Check sheet for the modelled part. Datum: model origin and axes. Units: mm. A direction names the side the tool comes from. Give positions to 0.01 mm unless a question says otherwise; leave off trailing zeros. Order: outer loops, then holes, each group sorted by start corner. A loop starts at its lowest first (then second) coordinate and runs counter-clockwise, first axis right, second up.
from build123d import *

# Parameters (mm, degrees)
F0_R     = 33
F1_DEPTH = 101.6
F2_R     = 26.5
F3_DEPTH = 76.2
F4_R     = 16
F5_DEPTH = 2
F6_R     = 6
F7_DEPTH = 26


with BuildPart() as f1:
    # F0 (on Right) → F1 (new body)
    with BuildSketch(Plane.YZ):
        Circle(F0_R)
    extrude(amount=F1_DEPTH)

    # F2 (on face) → F3 (join)
    with BuildSketch(Plane.YZ.offset(101.6)):
        Circle(F2_R)
    extrude(amount=F3_DEPTH)

    # F4 (on face) → F5 (join)
    with BuildSketch(Plane.YZ.offset(177.8)):
        Circle(F4_R)
    extrude(amount=F5_DEPTH)

    # F6 (on face) → F7 (join)
    with BuildSketch(Plane.YZ.offset(179.8)):
        Circle(F6_R)
    extrude(amount=F7_DEPTH)


solid = f1.part
1) Depth check by flat-ended pin: pin 1 Ø1.5 at (y, z) = (-22.5, 13) entering from +X; pin 2 Ø8 at (x, y) = (110, 3.5) entering from -Z; pin 3 Ø10 at (x, z) = (63, 18.5) entering from +Y. Enter the tip coordinate at first touch or a pass-through.
Recorded:
pin 1: stops at x = 177.8
pin 2: stops at z = -26.5
pin 3: stops at y = 30.11
2) Set-up check for faces 1 (the face through (139.167, 14.246, 22.345)), 2 (the face through (50.1, 30.5, -12.6)): record each of +Z, -Z, +X, -X, +Y, -Y from which the full face is reachable in a straight line by a thin tool's end or side.
Recorded:
face 1: +X
face 2: +X, -X
3) Section check A-A, the plane z = 0. Record the cut outline in (x, y), then the cut area to 3 significant figures.
Recorded:
outline: (0, -33) - (101.6, -33) - (101.6, -26.5) - (177.8, -26.5) - (177.8, -16) - (179.8, -16) - (179.8, -6) - (205.8, -6) - (205.8, 6) - (179.8, 6) - (179.8, 16) - (177.8, 16) - (177.8, 26.5) - (101.6, 26.5) - (101.6, 33) - (0, 33) - close
area: 11,100 mm2
4) Section check D-D, the plane y = -21. Record the cut outline in (x, z), then the cut area to 3 significant figures.
Recorded:
outline: (0, -25.46) - (101.6, -25.46) - (101.6, -16.16) - (177.8, -16.16) - (177.8, 16.16) - (101.6, 16.16) - (101.6, 25.46) - (0, 25.46) - close
area: 7,640 mm2
5) Material ranges on L1, parallel to X at y = 17.5, z = -1; L2, parallel to X at y = -1.5, z = 10.5; L3, parallel to Z at x = 69, y = 1, recorded low to high.
Recorded:
L1: x = 0 to 177.8
L2: x = 0 to 179.8
L3: z = -32.98 to 32.98
6) Section check C-C, the plane x = 125.5. Record the cut outline in (y, z), then the cut area to 3 significant figures.
Recorded:
outline: circle Ø53 at (0, 0)
area: 2,210 mm2
